Autodesk Inventor part; units mm, degrees
ref_plane "YZ Plane" through (0, 0, 0) normal (1, 0, 0) x (0, 1, 0)
ref_plane "XZ Plane" through (0, 0, 0) normal (0, 1, 0) x (-1, 0, 0)
ref_plane "XY Plane" through (0, 0, 0) normal (0, 0, 1) x (1, 0, 0)
sketch "Эскиз1" plane through (0, 0, 0) normal (0, 0, 1) x (1, 0, 0)
  line L0 (0, 0) -> (55.5, 0)
  line L1 (55.5, 0) -> (55.5, 6)
  line L2 (55.5, 6) -> (0, 6)
  line L3 (0, 6) -> (0, 0)
  line L4 (0, 6) -> (6, 6)
  line L5 (6, 6) -> (6, 11)
  line L6 (6, 11) -> (0, 11)
  line L7 (0, 11) -> (0, 6)
  line L8 (55.5, 6) -> (49.5, 6)
  line L9 (49.5, 6) -> (49.5, 38)
  line L10 (49.5, 38) -> (55.5, 38)
  line L11 (55.5, 38) -> (55.5, 6)
  dimension "d0" = 38
  dimension "d1" = 6
  dimension "d2" = 6
  dimension "d3" = 6
  dimension "d4" = 11
  dimension "d5" = 55.5
extrude "Выдавливание1" add sketch "Эскиз1" along normal blind 20.5
sketch "Эскиз2" plane through (55.5, 0, 0) normal (1, 0, 0) x (0, 0, -1)
  circle A0 centre (-10.25, 26.5) radius 4.5
  circle A1 centre (-10.25, 11.5) radius 4.5
  line L0 (-5.75, 26.5) -> (-5.75, 11.5)
  line L1 (-14.75, 26.5) -> (-14.75, 11.5)
  line L2 (0, 0) -> (-20.5, 0)
  point P0 (-10.25, 0)
  dimension "d8" = 9
  dimension "d9" = 11.5
  dimension "d10" = 24
extrude "Выдавливание2" cut sketch "Эскиз2" against normal up to next
sketch "Эскиз3" plane through (0, 0, 0) normal (0, -1, 0) x (1, 0, 0)
  circle A0 centre (37.5, 10.25) radius 2
  line L0 (55.5, 0) -> (55.5, 20.5)
  point P0 (0, 0)
  point P1 (55.5, 10.25)
  dimension "d13" = 4
  dimension "d14" = 18
extrude "Выдавливание3" cut sketch "Эскиз3" against normal up to next
sketch "Эскиз4" plane through (49.5, 38, 0) normal (0, 1, 0) x (1, 0, 0)
  circle A0 centre (3, -15.25) radius 1
  circle A1 centre (3, -5.25) radius 1
  line L0 (0, 0) -> (0, -20.5)
  line L1 (6, -20.5) -> (0, -20.5)
  line L2 (3, -5.25) -> (3, -15.25) construction
  line L3 (6, 0) -> (6, -20.5)
  point P0 (-49.5, 0)
  point P1 (3, -10.25)
  point P2 (6, -10.25)
  dimension "d17" = 2
  dimension "d18" = 10
  dimension "d19" = 2
extrude "Выдавливание4" cut sketch "Эскиз4" against normal blind 16
sketch "Эскиз5" plane through (0, 11, 0) normal (0, 1, 0) x (1, 0, 0)
  circle A0 centre (3, -5.25) radius 1.5
  circle A1 centre (3, -15.25) radius 1.5
  circle A2 centre (52.5, -5.25) radius 1
  circle A3 centre (52.5, -15.25) radius 1
  line L0 (6, 0) -> (0, 0)
  point P0 (3, 0)
  dimension "d23" = 3
extrude "Выдавливание5" cut sketch "Эскиз5" against normal up to next contours A0 | A1
properties part number "kreplenie1" material "Пластик АБС"
Check sheet for the modelled part. Datum: model origin and axes. Units: mm. A direction names the side the tool comes from. Round coordinates to 2 decimals unless told otherwise and drop trailing zeros. Loops run counter-clockwise (first coordinate to the right, second up) from the corner with the lowest first, then second, coordinate; pieces in that order, holes last. Notation, with made-up numbers: M 28,76.5 L 53,76.5 A25 cw 53,90.5 Z; hole C 72,57 d10. An arc over 180 degrees is marked long. One line per item, written item: value.
(1) Thickness scan on line 1 (Z direction, x = 3, y = 7); line 2 (X direction, y = 3.5, z = 5.25); line 3 (X direction, y = 7.5, z = 5.25). Record the ranges inside material, lowest first.
Computed values:
line 1: z = 0 to 3.75, 6.75 to 13.75, 16.75 to 20.5
line 2: x = 0 to 1.5, 4.5 to 55.5
line 3: x = 0 to 1.5, 4.5 to 6, 49.5 to 55.5
(2) Sectioned sample at D-D, the plane y = 14.5. Record the cut outline in (x, z).
Computed values:
outline: M 49.5,0 L 55.5,0 L 55.5,5.75 L 49.5,5.75 Z; M 49.5,14.75 L 55.5,14.75 L 55.5,20.5 L 49.5,20.5 Z
(3) Sectioned sample at A-A, the plane x = 37.5. Record the cut outline in (y, z), then the cut area to 3 significant figures.
Computed values:
outline: M 0,0 L 6,0 L 6,8.25 L 0,8.25 Z; M 0,12.25 L 6,12.25 L 6,20.5 L 0,20.5 Z
area: 99.0 mm^2
(4) Release check for a two-part mould opening along Y. For faces 1 (the face through (36.026, 2.958, 11.602)), 2 (the face through (53, 19, 5.75)), 3 (the face through (52, 22, 5)) record: +Y half, -Y half, draft (parallel to the pull), parting line (faces both ways), or undercut.
Computed values:
face 1: draft
face 2: undercut
face 3: +Y half
(5) Sectioned sample at C-C, the plane x = 3. Record the cut outline in (y, z), then the cut area to 4 significant figures.
Computed values:
outline: M 0,0 L 11,0 L 11,3.75 L 0,3.75 Z; M 0,6.75 L 11,6.75 L 11,13.75 L 0,13.75 Z; M 0,16.75 L 11,16.75 L 11,20.5 L 0,20.5 Z
area: 159.5 mm^2
(6) Depth check by flat-ended pin: pin 1 Ø2.5 at (x, z) = (3, 5.25) entering from +Y; pin 2 Ø1.8 at (x, z) = (4.5, 15) entering from +Y; pin 3 Ø1.5 at (x, z) = (20.5, 6.5) entering from +Y; pin 4 Ø1.5 at (y, z) = (8.5, 11) entering from +X. Enter the tip coordinate at first touch or a pass-through.
Computed values:
pin 1: passes through
pin 2: stops at y = 11
pin 3: stops at y = 6
pin 4: stops at x = 6
(7) Sectioned sample at B-B, the plane z = 10.25. Record the cut outline in (x, y).
Computed values:
outline: M 0,0 L 35.5,0 L 35.5,6 L 6,6 L 6,11 L 0,11 Z; M 39.5,0 L 55.5,0 L 55.5,7 L 49.5,7 L 49.5,6 L 39.5,6 Z; M 49.5,31 L 55.5,31 L 55.5,38 L 49.5,38 Z
(8) Access from +Z, -Z, +X, -X, +Y, -Y to the whole of each face (thin tool, end or side, straight path). Record for faces 4 (the face through (52.96, 30.11, 16.14)), 5 (the face through (28, 6, 10)), 6 (the face through (3, 11, 10)).
Computed values:
face 4: +Y
face 5: +Z, -Z, +Y
face 6: +Z, -Z, -X, +Y
